Source: CAD feature listing. Evaluate the final solid. Frame: model axes, mm. A direction names the side the tool comes from. Round coordinates to 2 decimals unless told otherwise and drop trailing zeros. Loops run counter-clockwise (first coordinate to the right, second up) from the corner with the lowest first, then second, coordinate; pieces in that order, holes last. Notation, with made-up numbers: M 15.5,-1 L 25.5,-1 A27 cw 25.5,32 Z; hole C 8.5,34.25 d1. An arc over 180 degrees is marked long. Answer as a JSON object with one key per item and string values.
from build123d import *

# Parameters (mm, degrees)
BOSS_EXTRUDE1_START = -1.8
SKETCH1_R           = 1
BOSS_EXTRUDE1_DEPTH = 1.8
BOSS_EXTRUDE2_START = -1.8
SKETCH1_5_R         = 1
SKETCH1_5_W         = 23.35
SKETCH1_5_H         = 12.5
SKETCH1_5_W_2       = 0.2
SKETCH1_5_H_2       = 11.7
BOSS_EXTRUDE2_DEPTH = 6.4
SKETCH1_6_R         = 1
CUT_EXTRUDE9_DEPTH  = 5.25
SKETCH6_R           = 1.25
BOSS_EXTRUDE4_DEPTH = 3
CUT_EXTRUDE6_START  = -8.2
SKETCH4_6_R         = 1.55
CUT_EXTRUDE6_DEPTH  = 5.2
BOSS_EXTRUDE3_DEPTH = 27.3
CUT_EXTRUDE7_START  = -3
SKETCH4_7_R         = 1.55
CUT_EXTRUDE7_DEPTH  = 30.3
CUT_EXTRUDE8_DEPTH  = 1.5


with BuildPart() as part:
    # Sketch1 → Boss-Extrude1 (new body)
    with BuildSketch(Plane.XZ.offset(10.394345176).offset(BOSS_EXTRUDE1_START)):
        Polygon((-30.246052812, 14.536068682), (-30.246052812, -0.963931318), (-25.671052812, -0.963931318), (-25.671052812, 11.536068682), (-2.321052812, 11.536068682), (-2.321052812, -0.963931318), (6.828947188, -0.963931318), (6.828947188, 11.536068682), (30.178947188, 11.536068682), (30.178947188, -0.963931318), (34.753947188, -0.963931318), (34.753947188, 14.536068682), align=None)
        with Locations((-27.871052812, 5.136068682)):
            Circle(SKETCH1_R, mode=Mode.SUBTRACT)
        with Locations((32.378947188, 5.136068682)):
            Circle(SKETCH1_R, mode=Mode.SUBTRACT)
    extrude(amount=BOSS_EXTRUDE1_DEPTH)

    # Sketch1_5 → Boss-Extrude2 (add)
    with BuildSketch(Plane.XZ.offset(10.394345176).offset(BOSS_EXTRUDE2_START)):
        with BuildLine():
            Line((-30.246052812, 14.536068682), (-30.246052812, -0.963931318))
            Line((-30.246052812, -0.963931318), (-25.671052812, -0.963931318))
            Line((-25.671052812, -0.963931318), (-25.671052812, -0.713931318))
            Line((-25.671052812, -0.713931318), (-29.746052812, -0.713931318))
            ThreePointArc((-29.746052812, -0.713931318), (-29.922829508, -0.640708013), (-29.996052812, -0.463931318))
            Line((-29.996052812, -0.463931318), (-29.996052812, 4.511068682))
            Line((-29.996052812, 4.511068682), (-28.651677562, 4.511068682))
            ThreePointArc((-28.651677562, 4.511068682), (-28.871052812, 5.136068682), (-28.651677562, 5.761068682))
            Line((-28.651677562, 5.761068682), (-29.996052812, 5.761068682))
            Line((-29.996052812, 5.761068682), (-29.996052812, 10.736068682))
            ThreePointArc((-29.996052812, 10.736068682), (-29.922829508, 10.912845377), (-29.746052812, 10.986068682))
            Line((-29.746052812, 10.986068682), (-25.671052812, 10.986068682))
            Line((-25.671052812, 10.986068682), (-25.671052812, 11.536068682))
            Line((-25.671052812, 11.536068682), (-2.321052812, 11.536068682))
            Line((-2.321052812, 11.536068682), (-2.321052812, -0.963931318))
            Line((-2.321052812, -0.963931318), (6.828947188, -0.963931318))
            Line((6.828947188, -0.963931318), (6.828947188, 11.536068682))
            Line((6.828947188, 11.536068682), (30.178947188, 11.536068682))
            Line((30.178947188, 11.536068682), (30.178947188, -0.963931318))
            Line((30.178947188, -0.963931318), (34.753947188, -0.963931318))
            Line((34.753947188, -0.963931318), (34.753947188, 14.536068682))
            Line((34.753947188, 14.536068682), (2.253947188, 14.536068682))
            Line((2.253947188, 14.536068682), (-30.246052812, 14.536068682))
        make_face()
        with Locations((-0.121052812, 5.136068682)):
            Circle(SKETCH1_5_R, mode=Mode.SUBTRACT)
        with Locations((4.628947188, 5.136068682)):
            Circle(SKETCH1_5_R, mode=Mode.SUBTRACT)
        with Locations((32.378947188, 5.136068682)):
            Circle(SKETCH1_5_R, mode=Mode.SUBTRACT)
        with Locations((18.503947188, 5.286068682)):
            Rectangle(SKETCH1_5_W, SKETCH1_5_H)
        with BuildLine():
            Line((19.103947188, 2.111068682), (18.425821266, 2.111068682))
            ThreePointArc((18.425821266, 2.111068682), (18.376229436, 2.097905601), (18.339693232, 2.06188169))
            ThreePointArc((18.339693232, 2.06188169), (7.078947188, 5.136068682), (18.339693232, 8.210255674))
            ThreePointArc((18.339693232, 8.210255674), (18.376229436, 8.174231764), (18.425821266, 8.161068682))
            Line((18.425821266, 8.161068682), (19.103947188, 8.161068682))
            ThreePointArc((19.103947188, 8.161068682), (22.128947188, 5.136068682), (19.103947188, 2.111068682))
        make_face(mode=Mode.SUBTRACT)
        Polygon((-25.671052812, -0.713931318), (-25.671052812, -0.963931318), (-2.321052812, -0.963931318), (-2.321052812, 11.536068682), (-25.671052812, 11.536068682), (-25.671052812, 10.986068682), (-25.471052812, 10.986068682), (-25.471052812, -0.713931318), align=None)
        with BuildLine():
            ThreePointArc((-13.831798857, 2.06188169), (-13.868335061, 2.097905601), (-13.917926891, 2.111068682))
            Line((-13.917926891, 2.111068682), (-14.596052812, 2.111068682))
            ThreePointArc((-14.596052812, 2.111068682), (-17.621052812, 5.136068682), (-14.596052812, 8.161068682))
            Line((-14.596052812, 8.161068682), (-13.917926891, 8.161068682))
            ThreePointArc((-13.917926891, 8.161068682), (-13.868335061, 8.174231764), (-13.831798857, 8.210255674))
            ThreePointArc((-13.831798857, 8.210255674), (-2.571052812, 5.136068682), (-13.831798857, 2.06188169))
        make_face(mode=Mode.SUBTRACT)
        with BuildLine():
            Line((-29.746052812, -0.713931318), (-25.671052812, -0.713931318))
            Line((-25.671052812, -0.713931318), (-25.671052812, 10.986068682))
            Line((-25.671052812, 10.986068682), (-29.746052812, 10.986068682))
            ThreePointArc((-29.746052812, 10.986068682), (-29.922829508, 10.912845377), (-29.996052812, 10.736068682))
            Line((-29.996052812, 10.736068682), (-29.996052812, 5.761068682))
            Line((-29.996052812, 5.761068682), (-28.651677562, 5.761068682))
            ThreePointArc((-28.651677562, 5.761068682), (-27.539861591, 6.079632339), (-26.871052812, 5.136068682))
            ThreePointArc((-26.871052812, 5.136068682), (-27.539861591, 4.192505025), (-28.651677562, 4.511068682))
            Line((-28.651677562, 4.511068682), (-29.996052812, 4.511068682))
            Line((-29.996052812, 4.511068682), (-29.996052812, -0.463931318))
            ThreePointArc((-29.996052812, -0.463931318), (-29.922829508, -0.640708013), (-29.746052812, -0.713931318))
        make_face()
        with Locations((-25.571052812, 5.136068682)):
            Rectangle(SKETCH1_5_W_2, SKETCH1_5_H_2)
        with Locations((4.628947188, 5.136068682)):
            Circle(SKETCH1_5_R)
        with Locations((-0.121052812, 5.136068682)):
            Circle(SKETCH1_5_R)
    extrude(amount=-BOSS_EXTRUDE2_DEPTH)

    # Sketch1_6 → Cut-Extrude9 (cut)
    with BuildSketch(Plane.XZ.offset(10.394345176)):
        with Locations((4.628947188, 5.136068682)):
            Circle(SKETCH1_6_R)
        with Locations((-0.121052812, 5.136068682)):
            Circle(SKETCH1_6_R)
    extrude(amount=-CUT_EXTRUDE9_DEPTH, mode=Mode.SUBTRACT)

    # Sketch6 → Boss-Extrude4 (add)
    with BuildSketch(Plane.XY.offset(14.536068682)):
        with BuildLine():
            Line((34.753947188, -10.394345176), (9.394953593, -10.394345176))
            ThreePointArc((9.394953593, -10.394345176), (23.644922083, -16.360870979), (29.392610104, -30.700505374))
            ThreePointArc((29.392610104, -30.700505374), (29.532392174, -31.049241035), (29.878947188, -31.194345176))
            Line((29.878947188, -31.194345176), (34.753947188, -31.194345176))
            Line((34.753947188, -31.194345176), (34.753947188, -10.394345176))
        make_face()
        with Locations((32.878947188, -26.30759383)):
            Circle(SKETCH6_R, mode=Mode.SUBTRACT)
        with Locations((32.878947188, -18.534091138)):
            Circle(SKETCH6_R, mode=Mode.SUBTRACT)
        with BuildLine():
            Line((-4.887059217, -10.394345176), (-30.246052812, -10.394345176))
            Line((-30.246052812, -10.394345176), (-30.246052812, -16.729871547))
            Line((-30.246052812, -16.729871547), (-28.371052812, -15.647339792))
            Line((-28.371052812, -15.647339792), (-25.871052812, -17.090715465))
            Line((-25.871052812, -17.090715465), (-25.871052812, -19.977466811))
            Line((-25.871052812, -19.977466811), (-28.371052812, -21.420842484))
            Line((-28.371052812, -21.420842484), (-30.246052812, -20.338310729))
            Line((-30.246052812, -20.338310729), (-30.246052812, -24.503374239))
            Line((-30.246052812, -24.503374239), (-28.371052812, -23.420842484))
            Line((-28.371052812, -23.420842484), (-25.871052812, -24.864218157))
            Line((-25.871052812, -24.864218157), (-25.871052812, -27.750969503))
            Line((-25.871052812, -27.750969503), (-28.371052812, -29.194345176))
            Line((-28.371052812, -29.194345176), (-30.246052812, -28.111813421))
            Line((-30.246052812, -28.111813421), (-30.246052812, -31.194345176))
            Line((-30.246052812, -31.194345176), (-25.371052812, -31.194345176))
            ThreePointArc((-25.371052812, -31.194345176), (-25.024497799, -31.049241035), (-24.884715729, -30.700505374))
            ThreePointArc((-24.884715729, -30.700505374), (-19.137027708, -16.360870979), (-4.887059217, -10.394345176))
        make_face()
        Polygon((-28.371052812, -23.420842484), (-30.246052812, -24.503374239), (-30.246052812, -28.111813421), (-28.371052812, -29.194345176), (-25.871052812, -27.750969503), (-25.871052812, -24.864218157), align=None)
        with Locations((-28.371052812, -26.30759383)):
            Circle(SKETCH6_R, mode=Mode.SUBTRACT)
        Polygon((-28.371052812, -15.647339792), (-30.246052812, -16.729871547), (-30.246052812, -20.338310729), (-28.371052812, -21.420842484), (-25.871052812, -19.977466811), (-25.871052812, -17.090715465), align=None)
        with Locations((-28.371052812, -18.534091138)):
            Circle(SKETCH6_R, mode=Mode.SUBTRACT)
    extrude(amount=-BOSS_EXTRUDE4_DEPTH)

    # Sketch4_6 → Cut-Extrude6 (cut)
    with BuildSketch(Plane(origin=(0, -2.194345176, 0), x_dir=(1, 0, 0), z_dir=(0, 1, 0)).offset(CUT_EXTRUDE6_START)):
        Polygon((5.103947188, -11.010607671), (5.103947188, -7.719711137), (2.253947188, -6.07426287), (-0.596052812, -7.719711137), (-0.596052812, -11.010607671), (2.253947188, -12.656055938), align=None)
        with Locations((2.253947188, -9.365159404)):
            Circle(SKETCH4_6_R, mode=Mode.SUBTRACT)
        with Locations((2.253947188, -9.365159404)):
            Circle(SKETCH4_6_R)
    extrude(amount=CUT_EXTRUDE6_DEPTH, mode=Mode.SUBTRACT)

    # Sketch4 → Boss-Extrude3 (add)
    with BuildSketch(Plane(origin=(0, -2.194345176, 0), x_dir=(1, 0, 0), z_dir=(0, 1, 0))):
        with BuildLine():
            Line((1.993192449, -13.656055938), (2.514701927, -13.656055938))
            ThreePointArc((2.514701927, -13.656055938), (6.217553798, -11.71318089), (6.722992999, -7.562228392))
            ThreePointArc((6.722992999, -7.562228392), (6.440270151, -3.658198764), (8.34156903, -0.236730934))
            ThreePointArc((8.34156903, -0.236730934), (8.500600778, 0.528068047), (7.852347904, 0.963931318))
            Line((7.852347904, 0.963931318), (-3.344453529, 0.963931318))
            ThreePointArc((-3.344453529, 0.963931318), (-3.992706402, 0.528068047), (-3.833674654, -0.236730934))
            ThreePointArc((-3.833674654, -0.236730934), (-1.932375775, -3.658198764), (-2.215098624, -7.562228392))
            ThreePointArc((-2.215098624, -7.562228392), (-1.709659423, -11.71318089), (1.993192449, -13.656055938))
        make_face()
    extrude(amount=BOSS_EXTRUDE3_DEPTH)

    # Sketch4_7 → Cut-Extrude7 (cut)
    with BuildSketch(Plane(origin=(0, -2.194345176, 0), x_dir=(1, 0, 0), z_dir=(0, 1, 0)).offset(CUT_EXTRUDE7_START)):
        with Locations((2.253947188, -9.365159404)):
            Circle(SKETCH4_7_R)
    extrude(amount=CUT_EXTRUDE7_DEPTH, mode=Mode.SUBTRACT)

    # Sketch5 → Cut-Extrude8 (cut)
    with BuildSketch(Plane(origin=(0, 25.105654824, 0), x_dir=(1, 0, 0), z_dir=(0, 1, 0))):
        Polygon((5.385896038, -6.427447361), (3.697691675, -4.382517944), (6.366164089, -1.150185498), (5.016629458, -0.036068682), (2.253947188, -3.382517944), (-0.508735082, -0.036068682), (-1.858269713, -1.150185498), (0.8102027, -4.382517944), (-0.878001663, -6.427447361), (0.471532968, -7.541564177), (2.253947188, -5.382517944), (4.036361407, -7.541564177), align=None)
    extrude(amount=-CUT_EXTRUDE8_DEPTH, mode=Mode.SUBTRACT)


solid = part.part
Item 1: Section A-A on y = -7. Return the cut outline in (x, z) (3 decimals), then the cut area to 3 significant figures.
Answer sheet:
{"outline": "M -30.246,-0.964 L 34.754,-0.964 L 34.754,14.536 L -30.246,14.536 Z; hole C -27.871,5.136 d2; hole M -14.596,2.111 L -13.918,2.111 A0.1 cw -13.832,2.062 A6.05 ccw long -13.832,8.21 A0.1 cw -13.918,8.161 L -14.596,8.161 A3.025 ccw Z; hole C -0.121,5.136 d2; hole M -0.596,7.72 L 2.254,6.074 L 5.104,7.72 L 5.104,11.011 L 2.254,12.656 L -0.596,11.011 Z; hole C 4.629,5.136 d2; hole M 18.34,2.062 A0.1 cw 18.426,2.111 L 19.104,2.111 A3.025 ccw 19.104,8.161 L 18.426,8.161 A0.1 cw 18.34,8.21 A6.05 ccw long Z; hole C 32.379,5.136 d2", "area": "706 mm²"}
Item 2: Section B-B on x = -10. Return the cut outline in (y, z), then the cut area to 3 significant figures.
Answer sheet:
{"outline": "M -11.06,11.54 L -8.59,11.54 L -8.59,11.03 L -2.19,11.03 L -2.19,14.54 L -11.06,14.54 Z; M -8.59,-0.96 L -2.19,-0.96 L -2.19,-0.75 L -8.59,-0.75 Z", "area": "31.2 mm²"}
Item 3: Section D-D on y = 10.5. Return the cut outline in (x, z).
Answer sheet:
{"outline": "M -3.83,0.24 A0.7 ccw -3.34,-0.96 L 7.85,-0.96 A0.7 ccw 8.34,0.24 A6.85 cw 6.72,7.56 A4.5 ccw 2.51,13.66 L 1.99,13.66 A4.5 ccw -2.22,7.56 A6.85 cw Z; hole C 2.25,9.37 d3.1"}
Item 4: Line query: probe 1 along Z at (x, y) = (-14, -4.5); probe 2 along X at (y, z) = (-2, 8); probe 3 along X at (y, z) = (-25.5, 12.25). Output: solid intervals per line, ascending. Write a range as from..to.
Answer sheet:
{"probe 1": "z = -0.96..2.11, 8.16..14.54", "probe 2": "x = -2.36..1.52, 2.99..6.86", "probe 3": "x = -30.25..-29.33, -27.42..-24.28, 28.79..31.92, 33.83..34.75"}
Item 5: Section C-C on y = -15.5. Return the cut outline in (x, z).
Answer sheet:
{"outline": "M -30.25,11.54 L -18.23,11.54 L -18.23,14.54 L -30.25,14.54 Z; M 22.74,11.54 L 34.75,11.54 L 34.75,14.54 L 22.74,14.54 Z"}
Item 6: Pull-direction query (X, two-part tool) for faces 6 (the flat face through (34.754, -10, 12)), 7 (the flat face through (-29, -10.394, 5.4)), 8 (the flat face through (-23, -17, 11.536)); classes: pulls with the +X half, pulls with the -X half, needs draft (parallel to the pull), parting line crosses it, or undercut.
Answer sheet:
{"face 6": "pulls with the +X half", "face 7": "needs draft", "face 8": "undercut"}
Item 7: Contact query for flat-ended pins moving along their axis: pin 1 Ø6 at (x, z) = (-18, 5.5) entering from +Y; pin 2 Ø11.5 at (x, y) = (-13.5, -18) entering from -Z; pin 3 Ø2.5 at (x, z) = (32.38, 5.14) entering from -Y. Output: stop coordinate, or through.
Answer sheet:
{"pin 1": "stops at y = -2.19", "pin 2": "stops at z = 11.54", "pin 3": "stops at y = -10.39"}
Item 8: Access query for faces 1 (the cylindrical face through (6, 11, 12)), 2 (the cylindrical face through (7.083, -5.439, 4.915)), 3 (the flat face through (5.01, 24.37, 2.79)), 4 (the cylindrical face through (-0.251, -7.806, 6.128)), 5 (the flat face through (2, -10, 14.536)). Directions: +Z, -Z, +X, -X, +Y, -Y. A direction counts if a zero-diameter tool reaches every point of the face in a straight line with its end or side. Return the directions, or none.
Answer sheet:
{"face 1": "+X, +Y", "face 2": "+Y, -Y", "face 3": "+Y", "face 4": "-Y", "face 5": "+Z, +X, -X, +Y, -Y"}
